```python
from build123d import *

# Parameters (mm, degrees)
SKETCH1_W           = 44
SKETCH1_H           = 44
BOSS_EXTRUDE1_DEPTH = 1.5
SKETCH1_3_W         = 42
SKETCH1_3_H         = 42
BOSS_EXTRUDE2_DEPTH = 3.8
BOSS_EXTRUDE3_START = 3.8
SKETCH1_5_W         = 44
SKETCH1_5_H         = 44
BOSS_EXTRUDE3_DEPTH = 1.5
BOSS_EXTRUDE4_START = 5.3
SKETCH1_6_W         = 31
SKETCH1_6_H         = 31
BOSS_EXTRUDE4_DEPTH = 2.3
BOSS_EXTRUDE5_START = 7.6
SKETCH1_7_W         = 33
SKETCH1_7_H         = 33
BOSS_EXTRUDE5_DEPTH = 1.5
BOSS_EXTRUDE6_START = 9.1
SKETCH1_8_W         = 20
SKETCH1_8_H         = 20
BOSS_EXTRUDE6_DEPTH = 2.3
BOSS_EXTRUDE7_START = 12.9
SKETCH1_12_W        = 22
SKETCH1_12_H        = 22
BOSS_EXTRUDE7_DEPTH = 1.5


with BuildPart() as part:
    # Sketch1 → Boss-Extrude1 (new body)
    with BuildSketch(Plane(origin=(0, 0, 0), x_dir=(1, 0, 0), z_dir=(0, 1, 0))):
        Rectangle(SKETCH1_W, SKETCH1_H)
    extrude(amount=BOSS_EXTRUDE1_DEPTH)

    # Sketch1<3> → Boss-Extrude2 (add)
    with BuildSketch(Plane(origin=(0, 0, 0), x_dir=(1, 0, 0), z_dir=(0, 1, 0))):
        Rectangle(SKETCH1_3_W, SKETCH1_3_H)
    extrude(amount=BOSS_EXTRUDE2_DEPTH)

    # Sketch1<5> → Boss-Extrude3 (add)
    with BuildSketch(Plane(origin=(0, 0, 0), x_dir=(1, 0, 0), z_dir=(0, 1, 0)).offset(BOSS_EXTRUDE3_START)):
        Rectangle(SKETCH1_5_W, SKETCH1_5_H)
    extrude(amount=BOSS_EXTRUDE3_DEPTH)

    # Sketch1<6> → Boss-Extrude4 (add)
    with BuildSketch(Plane(origin=(0, 0, 0), x_dir=(1, 0, 0), z_dir=(0, 1, 0)).offset(BOSS_EXTRUDE4_START)):
        Rectangle(SKETCH1_6_W, SKETCH1_6_H)
    extrude(amount=BOSS_EXTRUDE4_DEPTH)

    # Sketch1<7> → Boss-Extrude5 (add)
    with BuildSketch(Plane(origin=(0, 0, 0), x_dir=(1, 0, 0), z_dir=(0, 1, 0)).offset(BOSS_EXTRUDE5_START)):
        Rectangle(SKETCH1_7_W, SKETCH1_7_H)
    extrude(amount=BOSS_EXTRUDE5_DEPTH)

    # Sketch1<8> → Boss-Extrude6 (add)
    with BuildSketch(Plane(origin=(0, 0, 0), x_dir=(1, 0, 0), z_dir=(0, 1, 0)).offset(BOSS_EXTRUDE6_START)):
        Rectangle(SKETCH1_8_W, SKETCH1_8_H)
    extrude(amount=BOSS_EXTRUDE6_DEPTH)

    # Sketch1<12> → Boss-Extrude7 (add)
    with BuildSketch(Plane(origin=(0, 0, 0), x_dir=(1, 0, 0), z_dir=(0, 1, 0)).offset(BOSS_EXTRUDE7_START)):
        Rectangle(SKETCH1_12_W, SKETCH1_12_H)
    extrude(amount=-BOSS_EXTRUDE7_DEPTH)


solid = part.part
```
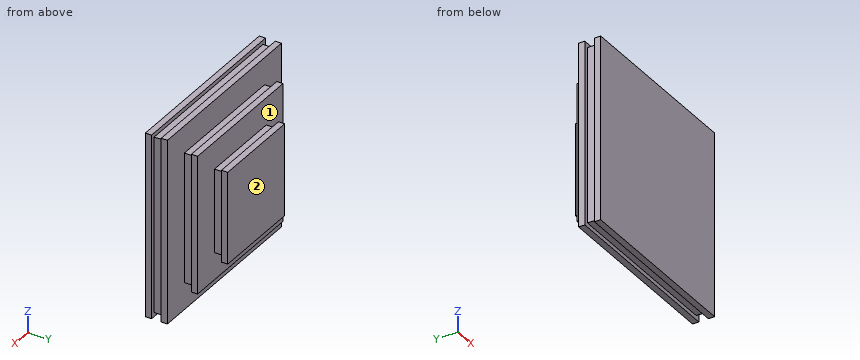
Work out the finished part from the listing and answer in its coordinate system (mm). Face numbers are marked on the shaded views. A direction names the side the tool comes from. Round coordinates to 2 decimals unless told otherwise and drop trailing zeros. Write each loop counter-clockwise with the first axis right and the second up, starting at its lowest first coordinate (ties: lowest second). Pieces come first, ordered by that corner, then holes.
1) A cutting plane is placed at D-D on z = -14. Determine the outline of the cut face in (x, y).
2) A cutting plane is placed at B-B on z = 2. Determine the outline of the cut face in (x, y).
3) Flat-ended cylindrical pins translate along their axes: P1, Ø5, axis at x = -4.5, y = 11, coming from the -Z side; P2, Ø1.1, axis at x = -4, y = 10, coming from the +Z side; P3, Ø0.8, axis at y = 12, z = -4.5, coming from the +X side. Find the tip coordinate at first contact, or state that the pin passes through.
4) A cutting plane is placed at C-C on y = 12. Determine the outline of the cut face in (x, z).
5) Consider probe 1 along Z at (x, y) = (-8, 11.5); probe 2 along Z at (x, y) = (9, 10); probe 3 along Y at (x, z) = (-20, 4). Determine where each line is inside the solid, lowest interval first.
6) A cutting plane is placed at A-A on x = 8.5. Determine the outline of the cut face in (y, z).
7) Which of the six approach directions +Z, -Z, +X, -X, +Y, -Y give full straight-line access (tool end or side, diameter ignored) to the marked faces 1 and 2?
Entries:
1. outline: (-22, 0) - (22, 0) - (22, 1.5) - (21, 1.5) - (21, 3.8) - (22, 3.8) - (22, 5.3) - (15.5, 5.3) - (15.5, 7.6) - (16.5, 7.6) - (16.5, 9.1) - (-16.5, 9.1) - (-16.5, 7.6) - (-15.5, 7.6) - (-15.5, 5.3) - (-22, 5.3) - (-22, 3.8) - (-21, 3.8) - (-21, 1.5) - (-22, 1.5) - close
2. outline: (-22, 0) - (22, 0) - (22, 1.5) - (21, 1.5) - (21, 3.8) - (22, 3.8) - (22, 5.3) - (15.5, 5.3) - (15.5, 7.6) - (16.5, 7.6) - (16.5, 9.1) - (10, 9.1) - (10, 11.4) - (11, 11.4) - (11, 12.9) - (-11, 12.9) - (-11, 11.4) - (-10, 11.4) - (-10, 9.1) - (-16.5, 9.1) - (-16.5, 7.6) - (-15.5, 7.6) - (-15.5, 5.3) - (-22, 5.3) - (-22, 3.8) - (-21, 3.8) - (-21, 1.5) - (-22, 1.5) - close
3. P1: stops at z = -16.5
3. P2: stops at z = 10
3. P3: stops at x = 11
4. outline: (-11, -11) - (11, -11) - (11, 11) - (-11, 11) - close
5. probe 1: z = -11 to 11
5. probe 2: z = -10 to 10
5. probe 3: y = 0 to 5.3
6. outline: (0, -22) - (1.5, -22) - (1.5, -21) - (3.8, -21) - (3.8, -22) - (5.3, -22) - (5.3, -15.5) - (7.6, -15.5) - (7.6, -16.5) - (9.1, -16.5) - (9.1, -10) - (11.4, -10) - (11.4, -11) - (12.9, -11) - (12.9, 11) - (11.4, 11) - (11.4, 10) - (9.1, 10) - (9.1, 16.5) - (7.6, 16.5) - (7.6, 15.5) - (5.3, 15.5) - (5.3, 22) - (3.8, 22) - (3.8, 21) - (1.5, 21) - (1.5, 22) - (0, 22) - close
7. face 1: none
7. face 2: +Z, -Z, +X, -X, +Y
